The model under review builds one solid part; all positions refer to its coordinate system, in mm. Round coordinates to 2 decimals unless told otherwise and drop trailing zeros. Loops run counter-clockwise (first coordinate to the right, second up) from the corner with the lowest first, then second, coordinate; pieces in that order, holes last. Notation, with made-up numbers: M 45.5,-38.5 L 49.5,-38.5 A16 ccw 49.5,-25.5 Z; hole C -24.75,72.25 d4. An arc over 180 degrees is marked long. Use a Markdown table: item, result. Add a question column.
```python
from build123d import *

# Parameters (mm, degrees)
SKETCH1_W           = 148.5
SKETCH1_H           = 35
BOSS_EXTRUDE1_DEPTH = 3


with BuildPart() as part:
    # Sketch1 → Boss-Extrude1 (new body)
    with BuildSketch(Plane(origin=(0, 0, 0), x_dir=(1, 0, 0), z_dir=(0, 1, 0))):
        Polygon((0, 105), (0, 120), (-91.75, 120), (-91.75, 105), (-74.25, 105), align=None)
        Polygon((91.75, 105), (91.75, 120), (0, 120), (0, 105), (74.25, 105), align=None)
        Polygon((109.25, -105), (109.25, 120), (91.75, 120), (91.75, 105), (91.75, -105), align=None)
        Polygon((-91.75, 105), (-91.75, 120), (-109.25, 120), (-109.25, -105), (-91.75, -105), align=None)
        with BuildLine():
            Line((-109.25, -140), (-74.25, -140))
            Line((-74.25, -140), (-74.25, -105))
            Line((-74.25, -105), (-89.982233047, -120.732233047))
            ThreePointArc((-89.982233047, -120.732233047), (-89.440301169, -121.543291419), (-89.25, -122.5))
            ThreePointArc((-89.25, -122.5), (-90.793291419, -124.809698831), (-93.517766953, -124.267766953))
            Line((-93.517766953, -124.267766953), (-109.25, -140))
        make_face()
        with BuildLine():
            Line((-89.982233047, -120.732233047), (-74.25, -105))
            Line((-74.25, -105), (-91.75, -105))
            Line((-91.75, -105), (-109.25, -105))
            Line((-109.25, -105), (-109.25, -140))
            Line((-109.25, -140), (-93.517766953, -124.267766953))
            ThreePointArc((-93.517766953, -124.267766953), (-93.517766953, -120.732233047), (-89.982233047, -120.732233047))
        make_face()
        with Locations((0, -122.5)):
            Rectangle(SKETCH1_W, SKETCH1_H)
        with BuildLine():
            Line((74.25, -140), (109.25, -140))
            Line((109.25, -140), (93.517766953, -124.267766953))
            ThreePointArc((93.517766953, -124.267766953), (89.982233047, -124.267766953), (89.982233047, -120.732233047))
            Line((89.982233047, -120.732233047), (74.25, -105))
            Line((74.25, -105), (74.25, -140))
        make_face()
        with BuildLine():
            Line((109.25, -140), (109.25, -105))
            Line((109.25, -105), (91.75, -105))
            Line((91.75, -105), (74.25, -105))
            Line((74.25, -105), (89.982233047, -120.732233047))
            ThreePointArc((89.982233047, -120.732233047), (92.706708581, -120.190301169), (94.25, -122.5))
            ThreePointArc((94.25, -122.5), (94.059698831, -123.456708581), (93.517766953, -124.267766953))
            Line((93.517766953, -124.267766953), (109.25, -140))
        make_face()
    extrude(amount=BOSS_EXTRUDE1_DEPTH)


solid = part.part
```
(1) To check wall thickness, follow probe 1 along Z at (x, y) = (15, 1.45); probe 2 along X at (y, z) = (0.75, -60); probe 3 along Z at (x, y) = (91, 0.3). State the ranges of each line that lie inside material, in increasing order.
(2) Consider section A-A, the plane x = 11. Give the boundary of the cut face in (y, z).
(3) Consider section C-C, the plane z = 90.5. Give the boundary of the cut face in (x, y).
(4) Consider section B-B, the plane y = 1.1. Give the boundary of the cut face in (x, z).
Found:
| question | item | result |
|---|---|---|
| 1 | probe 1 | z = -120 to -105, 105 to 140 |
| 1 | probe 2 | x = -109.25 to -91.75, 91.75 to 109.25 |
| 1 | probe 3 | z = -120 to -105, 105 to 120.12, 124.88 to 140 |
| 2 | outline | M 0,-120 L 3,-120 L 3,-105 L 0,-105 Z; M 0,105 L 3,105 L 3,140 L 0,140 Z |
| 3 | outline | M -109.25,0 L -91.75,0 L -91.75,3 L -109.25,3 Z; M 91.75,0 L 109.25,0 L 109.25,3 L 91.75,3 Z |
| 4 | outline | M -109.25,-120 L 109.25,-120 L 109.25,140 L -109.25,140 Z; hole C -91.75,122.5 d5; hole M -91.75,-105 L 91.75,-105 L 91.75,105 L -91.75,105 Z; hole C 91.75,122.5 d5 |
